from build123d import *

# Parameters (mm, degrees)
SKETCH2_R               = 4
BOSS_EXTRUDE1_DEPTH     = 22
CHAMFER1_SIZE           = 0.9375
CUT_EXTRUDE1_DEPTH      = 3.95
CUT_EXTRUDE3_DEPTH      = 26.325793682
CUT_EXTRUDE3_DEPTH_BACK = 26.325793682
SKETCH11_R              = 0.79375


with BuildPart() as part:
    # Sketch2 → Boss-Extrude1 (new body)
    with BuildSketch(Plane(origin=(17.5, 0, 0), x_dir=(0, 0, -1), z_dir=(1, 0, 0))):
        Circle(SKETCH2_R)
    extrude(amount=-BOSS_EXTRUDE1_DEPTH)

    # Chamfer1
    chamfer1_edges = [part.edges().sort_by_distance(p)[0] for p in [
        (17.5, 0, 4),
    ]]
    chamfer(chamfer1_edges, length=CHAMFER1_SIZE)

    # Sketch10 → Revolve2 (revolve)
    with BuildSketch(Plane.XY, mode=Mode.PRIVATE) as revolve2_sk:
        Polygon((-2.190598923, 0), (-4.5, 4), (-17.5, 4), (-17.5, 0), align=None)
    revolve(revolve2_sk.sketch.rotate(Axis((-17.5, 0, 0), (1, 0, 0)), 270), axis=Axis((-17.5, 0, 0), (1, 0, 0)))

    # Sketch6 → Revolve1 (revolve)
    with BuildSketch(Plane.XY):
        Polygon((-21.875, 6.5), (-22.5, 5.875), (-22.5, 0), (-17.5, 0), (-17.5, 6.5), align=None)
    revolve(axis=Axis((-17.5, 0, 0), (-1, 0, 0)))

    # Sketch4 → Cut-Extrude1 (cut)
    with BuildSketch(Plane(origin=(-22.5, 0, 0), x_dir=(0, 0, -1), z_dir=(1, 0, 0))):
        Polygon((0, 2.886751346), (-2.5, 1.443375673), (-2.5, -1.443375673), (0, -2.886751346), (2.5, -1.443375673), (2.5, 1.443375673), align=None)
    extrude(amount=CUT_EXTRUDE1_DEPTH, mode=Mode.SUBTRACT)

    # Cut-Extrude2 cone 1 section (through the dimple's axis) → Cut-Extrude2 (revolve, cut)
    with BuildSketch(Plane(origin=(-22.5, 0, 0), x_dir=(0, 0, 1), z_dir=(0, 1, 0))):
        Polygon((0, 0), (2.886751346, 0), (0, 2.886751346), align=None)
    revolve(axis=Axis((-22.5, 0, 0), (1, 0, 0)), mode=Mode.SUBTRACT)

    # Sketch11 → Cut-Extrude3 (cut, two sides: drawn at the far end of the back side and taken through both)
    with BuildSketch(Plane(origin=(0, 2.165063509, -1.25), x_dir=(1, 0, 0), z_dir=(0, -0.8660254037844387, 0.49999999999999994)).offset(-CUT_EXTRUDE3_DEPTH_BACK)):
        with Locations(Location((-20.331624369, 0, 0), (0, 0, 270))):
            Circle(SKETCH11_R)
    extrude(amount=CUT_EXTRUDE3_DEPTH + CUT_EXTRUDE3_DEPTH_BACK, mode=Mode.SUBTRACT)


solid = part.part
Model file for the job. Use its own axes, mm. A direction names the side the tool comes from. Give positions to 0.01 mm unless a question says otherwise; leave off trailing zeros. Write each loop counter-clockwise with the first axis right and the second up, starting at its lowest first coordinate (ties: lowest second). Pieces come first, ordered by that corner, then holes. Notation, with made-up numbers: M 31.25,56.5 L 66.25,56.5 A22 ccw 66.25,87.5 Z; hole C -39,-9.5 d5. An arc over 180 degrees is marked long. One line per item, written item: value. Start each with the question number.
Q1. Probe probe 1 along X at (y, z) = (2.5, -5); probe 2 along X at (y, z) = (-2, -0.5); probe 3 along Z at (x, y) = (-20.5, -1.75). List the from-to ranges inside material, lowest first. Write a range as [from, to].
Q2. Saw through at B-B, the plane x = -13. Write the cut outline in (y, z).
Q3. Two-plate mould, pull along X, no slides. Class faces 4 (the cylindrical face through (-19.545, -3.821, 2.325)), 5 (the flat face through (-20.553, -1.674, 2.101)), 6 (the flat face through (-18.55, 0, 0)): +X half, -X half, draft (parallel to the pull), parting line (faces both ways), or undercut.
Q4. Drop flat-ended pins along their axis: pin 1 Ø3 at (x, z) = (9.5, 3.5) entering from -Y; pin 2 Ø5 at (x, z) = (-0.5, -1) entering from +Y; pin 3 Ø1.5 at (x, z) = (1, 3.5) entering from +Y. Give the stop position or say it passes through.
Q5. 3-axis set-ups, long thin cutter, end or side, ignore diameter. For faces 1 (the cylindrical face through (-0.707, -3.905, 0.867)), 2 (the conical face through (-22.304, 2.34, 1.328)), 3 (the flat face through (-22.5, -3, 1)): which of +Z, -Z, +X, -X, +Y, -Y reach the whole face in a straight line?
Output values:
1. probe 1: x = [-22.5, -17.5]
1. probe 2: x = [-18.55, 17.5]
1. probe 3: z = [-6.26, -1.97], [1.97, 6.26]
2. outline: C 0,0 d8
3. face 4: undercut
3. face 5: draft
3. face 6: -X half
4. pin 1: stops at y = -3.46
4. pin 2: stops at y = 4
4. pin 3: stops at y = 2.9
5. face 1: +X
5. face 2: -X
5. face 3: +Z, -Z, -X, +Y, -Y
